Check sheet for the modelled part. Datum: model origin and axes. Units: mm. A direction names the side the tool comes from. Round coordinates to 2 decimals unless told otherwise and drop trailing zeros. Order: outer loops, then holes, each group sorted by start corner. A loop starts at its lowest first (then second) coordinate and runs counter-clockwise, first axis right, second up. Notation, with made-up numbers: (38, 29.25) -> (73, 29.25) arc R9 ccw to (73, 42.25) -> close; hole circle Ø5 at (81, 56). An arc over 180 degrees is marked (long way). Answer in a Markdown table with one row per item.
from build123d import *

# Parameters (mm, degrees)
SKETCH1_R           = 2.55
SKETCH1_R_2         = 2.5
SKETCH1_R_3         = 10
BOSS_EXTRUDE1_DEPTH = 6.35


with BuildPart() as part:
    # Sketch1 → Boss-Extrude1 (new body)
    with BuildSketch(Plane(origin=(0, 0, 0), x_dir=(1, 0, 0), z_dir=(0, 1, 0))):
        with BuildLine():
            ThreePointArc((-147, 42.5), (-189.5, 0), (-147, -42.5))
            Line((-147, -42.5), (0, -42.5))
            ThreePointArc((0, -42.5), (42.5, 0), (0, 42.5))
            Line((0, 42.5), (-147, 42.5))
        make_face()
        with BuildLine():
            Line((-122, 2.55), (-102, 2.55))
            ThreePointArc((-102, 2.55), (-99.45, 0), (-102, -2.55))
            Line((-102, -2.55), (-122, -2.55))
            ThreePointArc((-122, -2.55), (-124.55, 0), (-122, 2.55))
        make_face(mode=Mode.SUBTRACT)
        with Locations(Location((-147, -37.5, 0), (0, 0, 270))):
            Circle(SKETCH1_R, mode=Mode.SUBTRACT)
        with BuildLine():
            ThreePointArc((-147, -27.55), (-149.55, -25), (-147, -22.45))
            Line((-147, -22.45), (-137, -22.45))
            ThreePointArc((-137, -22.45), (-134.45, -25), (-137, -27.55))
            Line((-137, -27.55), (-147, -27.55))
        make_face(mode=Mode.SUBTRACT)
        with Locations(Location((-184.5, 0, 0), (0, 0, 270))):
            Circle(SKETCH1_R, mode=Mode.SUBTRACT)
        with BuildLine():
            ThreePointArc((-172, -2.55), (-174.55, 0), (-172, 2.55))
            Line((-172, 2.55), (-162, 2.55))
            ThreePointArc((-162, 2.55), (-159.45, 0), (-162, -2.55))
            Line((-162, -2.55), (-172, -2.55))
        make_face(mode=Mode.SUBTRACT)
        with BuildLine():
            ThreePointArc((-147, -10), (-157, 0), (-147, 10))
            Line((-147, 10), (-137, 10))
            ThreePointArc((-137, 10), (-127, 0), (-137, -10))
            Line((-137, -10), (-147, -10))
        make_face(mode=Mode.SUBTRACT)
        with BuildLine():
            ThreePointArc((-147, 22.45), (-149.55, 25), (-147, 27.55))
            Line((-147, 27.55), (-137, 27.55))
            ThreePointArc((-137, 27.55), (-134.45, 25), (-137, 22.45))
            Line((-137, 22.45), (-147, 22.45))
        make_face(mode=Mode.SUBTRACT)
        with Locations(Location((-147, 37.5, 0), (0, 0, 270))):
            Circle(SKETCH1_R, mode=Mode.SUBTRACT)
        with Locations(Location((-73.5, 0, 0), (0, 0, 270))):
            Circle(SKETCH1_R, mode=Mode.SUBTRACT)
        with Locations(Location((-53.5, 0, 0), (0, 0, 270))):
            Circle(SKETCH1_R, mode=Mode.SUBTRACT)
        with Locations(Location((-93.5, 0, 0), (0, 0, 270))):
            Circle(SKETCH1_R, mode=Mode.SUBTRACT)
        with Locations(Location((0, 37.5, 0), (0, 0, 270))):
            Circle(SKETCH1_R, mode=Mode.SUBTRACT)
        with Locations(Location((0, -37.5, 0), (0, 0, 270))):
            Circle(SKETCH1_R, mode=Mode.SUBTRACT)
        with Locations(Location((-17.67766953, -17.67766953, 0), (0, 0, 270))):
            Circle(SKETCH1_R_2, mode=Mode.SUBTRACT)
        with Locations(Location((17.67766953, -17.67766953, 0), (0, 0, 270))):
            Circle(SKETCH1_R_2, mode=Mode.SUBTRACT)
        with Locations(Location((-17.67766953, 17.67766953, 0), (0, 0, 270))):
            Circle(SKETCH1_R_2, mode=Mode.SUBTRACT)
        with Locations(Location((0, 0, 0), (0, 0, 270))):
            Circle(SKETCH1_R_3, mode=Mode.SUBTRACT)
        with Locations(Location((37.5, 0, 0), (0, 0, 270))):
            Circle(SKETCH1_R, mode=Mode.SUBTRACT)
        with Locations(Location((17.67766953, 17.67766953, 0), (0, 0, 270))):
            Circle(SKETCH1_R_2, mode=Mode.SUBTRACT)
    extrude(amount=-BOSS_EXTRUDE1_DEPTH)


solid = part.part
Item 1: Depth check by flat-ended pin: P1, Ø4.5, axis at x = -17.68, z = 17.68, coming from the -Y side; P2, Ø3, axis at x = -166, y = -3.5, coming from the +Z side. Enter the tip coordinate at first touch or a pass-through.
Result sheet:
| item | result |
|---|---|
| P1 | passes through |
| P2 | stops at z = 38.73 |
Item 2: Cross-section at A-A (z = -37.5). Record the boundary of the cut face in (x, y), and give its area (3 significant figures).
Result sheet:
| item | result |
|---|---|
| outline | (-167, -6.35) -> (-149.55, -6.35) -> (-149.55, 0) -> (-167, 0) -> close; (-144.45, -6.35) -> (-2.55, -6.35) -> (-2.55, 0) -> (-144.45, 0) -> close; (2.55, -6.35) -> (20, -6.35) -> (20, 0) -> (2.55, 0) -> close |
| area | 1,120 mm^2 |
Item 3: Scan lines: line 1 (X direction, y = -4, z = -7); line 2 (Z direction, x = -103, y = -1); line 3 (X direction, y = -2.75, z = 6). Record each from-to range of solid material in increasing order. Write a range as [from, to].
Result sheet:
| item | result |
|---|---|
| line 1 | x = [-188.92, -154.14], [-129.86, -7.14], [7.14, 41.92] |
| line 2 | z = [-42.5, -2.55], [2.55, 42.5] |
| line 3 | x = [-189.07, -155], [-129, -8], [8, 42.07] |
Item 4: Cross-section at C-C (z = 25). Record the boundary of the cut face in (x, y).
Result sheet:
| item | result |
|---|---|
| outline | (-181.37, -6.35) -> (-149.55, -6.35) -> (-149.55, 0) -> (-181.37, 0) -> close; (-134.45, -6.35) -> (34.37, -6.35) -> (34.37, 0) -> (-134.45, 0) -> close |
Item 5: Cross-section at B-B (x = 37.5). Record the boundary of the cut face in (y, z).
Result sheet:
| item | result |
|---|---|
| outline | (-6.35, -20) -> (0, -20) -> (0, -2.55) -> (-6.35, -2.55) -> close; (-6.35, 2.55) -> (0, 2.55) -> (0, 20) -> (-6.35, 20) -> close |
Item 6: Mould release check, pull along Z, two halves, no side actions. Record for faces 3 (the flat face through (-75, 0, 9)), 4 (the cylindrical face through (-50.97, -3.13, -0.33)), 5 (the flat face through (-72, -3, -42.5)): pulls with the +Z half, pulls with the -Z half, needs draft (parallel to the pull), parting line crosses it, or undercut.
Result sheet:
| item | result |
|---|---|
| face 3 | needs draft |
| face 4 | undercut |
| face 5 | pulls with the -Z half |
Item 7: Cross-section at D-D (y = -3.75). State how many separate pieces and enclosed holes the cut face has, and give its area (3 significant figures).
Result sheet:
| item | result |
|---|---|
| separate pieces | 1 |
| enclosed holes | 19 |
| area | 16,700 mm^2 |
Item 8: Set-up check for faces 1 (the flat face through (-75, -6.35, 9)), 2 (the cylindrical face through (-157, -3, 0)): record each of +Z, -Z, +X, -X, +Y, -Y from which the full face is reachable in a straight line by a thin tool's end or side.
Result sheet:
| item | result |
|---|---|
| face 1 | +Z, -Z, +X, -X, -Y |
| face 2 | +Y, -Y |
